Can you work these out from the drawing? Everything is in mm from the part's minimum corner. Coordinates: 2 decimals unless noted, no trailing zeros. Loops run counter-clockwise (first coordinate to the right, second up) from the corner with the lowest first, then second, coordinate; pieces in that order, holes last. Notation, with made-up numbers: M 63.5,35.25 L 78.5,35.25 A29 cw 78.5,55.25 Z; hole C 9.25,-39.5 d4. An arc over 180 degrees is marked long. Use CSV: the item, a comma, the result in double quotes. Start each with the question number.
Q1. If we mould it in two halves opening along X, with no side actions, what happens to the marked faces 1, 2 and 3? For each: +X half, -X half, draft (parallel to the pull), parting line (faces both ways), or undercut.
Q2. If we section it at B-B (z = 7.25): Please give me the cut outline in (x, y).
Q3. If we section it at A-A (x = 7.25): Please give me the cut outline in (y, z), and give its area (3 significant figures).
Q4. Please list where these lines run through material, in increasing order: probe 1 along X at (y, z) = (1.75, 7.75); probe 2 along Z at (x, y) = (9, 2). Write a range as [from, to].
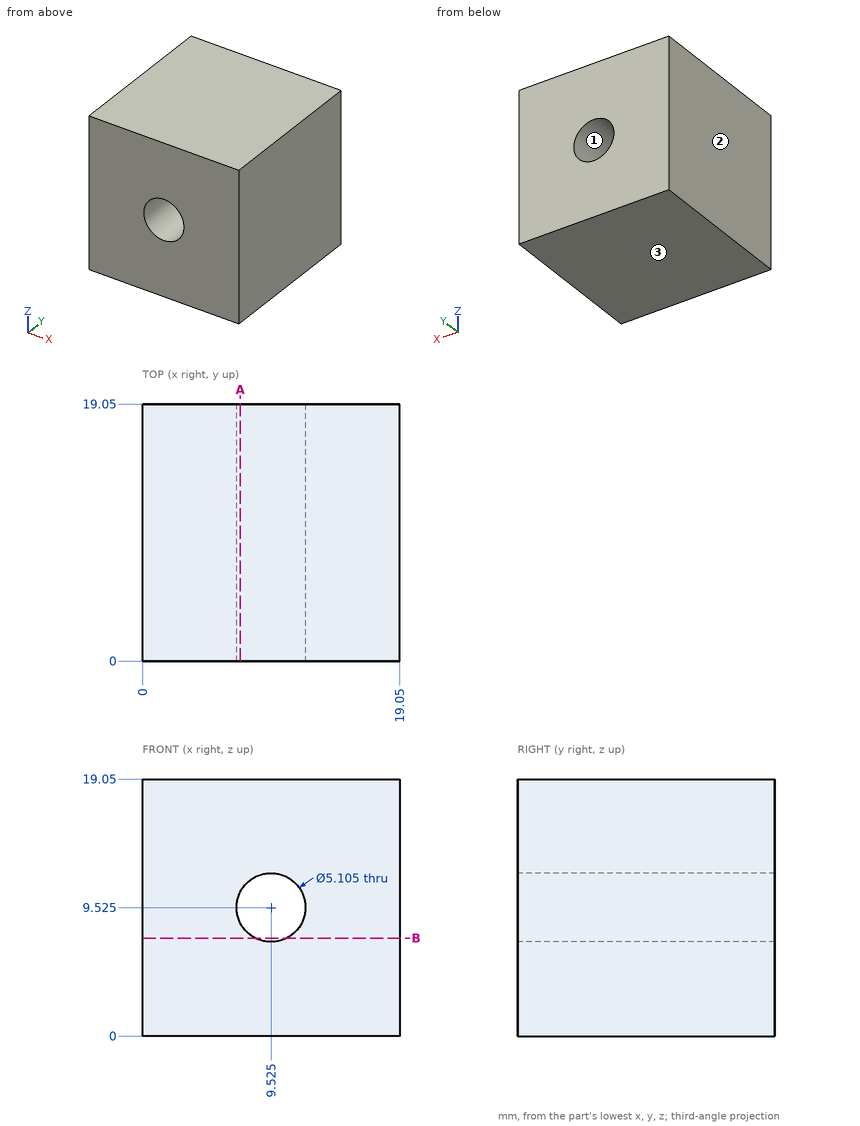
Results below:
1,face 1,"undercut"
1,face 2,"-X half"
1,face 3,"draft"
2,outline,"M 0,0 L 8.37,0 L 8.37,19.05 L 0,19.05 Z; M 10.68,0 L 19.05,0 L 19.05,19.05 L 10.68,19.05 Z"
3,outline,"M 0,0 L 19.05,0 L 19.05,8.37 L 0,8.37 Z; M 0,10.68 L 19.05,10.68 L 19.05,19.05 L 0,19.05 Z"
3,area,"319 mm^2"
4,probe 1,"[0, 7.69], [11.36, 19.05]"
4,probe 2,"[0, 7.03], [12.02, 19.05]"
